```python
from build123d import *

# Parameters (mm, degrees)
F0_W     = 11
F0_H     = 21
F1_DEPTH = 670
F2_W     = 5
F2_H     = 15
F3_DEPTH = 670
F4_W     = 10.772688
F4_H     = 2.595666
F4_H_2   = 2.404334
F5_DEPTH = 670


with BuildPart() as f1:
    # F0 (on Top) → F1 (new body)
    with BuildSketch(Plane.XY):
        Rectangle(F0_W, F0_H)
    extrude(amount=F1_DEPTH)

    # F2 (on face) → F3 (cut)
    with BuildSketch(Plane.XY.offset(670)):
        Rectangle(F2_W, F2_H)
    extrude(amount=-F3_DEPTH, mode=Mode.SUBTRACT)

    # F4 (on face) → F5 (cut)
    with BuildSketch(Plane.XY.offset(670)):
        with Locations((5.386344, 1.297833)):
            Rectangle(F4_W, F4_H)
        with Locations((5.386344, -1.202167)):
            Rectangle(F4_W, F4_H_2)
    extrude(amount=-F5_DEPTH, mode=Mode.SUBTRACT)


solid = f1.part
```
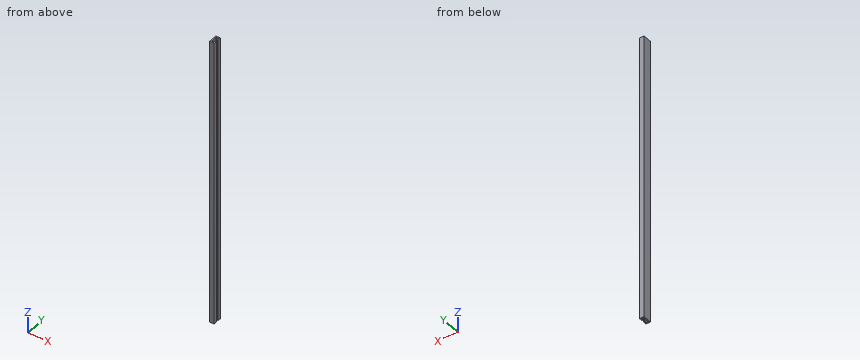
CAD build for the part. Positions are in the model's coordinates, mm. Coordinates: 2 decimals unless noted, no trailing zeros. Loops run counter-clockwise (first coordinate to the right, second up) from the corner with the lowest first, then second, coordinate; pieces in that order, holes last. Notation, with made-up numbers: (9.25, 87) - (46.25, 87) arc R23 ccw to (46.25, 104) - close; hole circle Ø5 at (43, -4). An arc over 180 degrees is marked (long way). Use CSV: the item, a comma, the result in double quotes. Start each with the question number.
Q1. Probe probe 1 along Y at (x, z) = (-1.25, 66.5); probe 2 along Y at (x, z) = (5.25, 84.5); probe 3 along X at (y, z) = (4.25, 344). List the from-to ranges inside material, lowest first. Write a range as from..to.
Q2. Cut at A-A, the plane x = -0.5. List the corners of the cut face in (y, z), then the cut area to 3 significant figures.
Q3. Cut at B-B, the plane z = 209.5. List the corners of the cut face in (x, y), then the cut area to 3 significant figures.
Q4. Drop a flat-ended pin along its axis: P1, Ø3, axis at y = 1, z = 248, coming from the +X side. Give the stop position or say it passes through.
Here are the results:
1,probe 1,"-10.5..-7.5, 7.5..10.5"
1,probe 2,"-10.5..-2.4, 2.6..10.5"
1,probe 3,"-5.5..-2.5, 2.5..5.5"
2,outline,"(-10.5, 0) - (-7.5, 0) - (-7.5, 670) - (-10.5, 670) - close; (7.5, 0) - (10.5, 0) - (10.5, 670) - (7.5, 670) - close"
2,area,"4,020 mm2"
3,outline,"(-5.5, -10.5) - (5.5, -10.5) - (5.5, -2.4) - (2.5, -2.4) - (2.5, -7.5) - (-2.5, -7.5) - (-2.5, 7.5) - (2.5, 7.5) - (2.5, 2.6) - (5.5, 2.6) - (5.5, 10.5) - (-5.5, 10.5) - close"
3,area,"141 mm2"
4,P1,"x = -2.5"
